Geometry: final body of the model. Coordinates: model frame, mm. A direction names the side the tool comes from. Give positions to 0.01 mm unless a question says otherwise; leave off trailing zeros. Loops run counter-clockwise (first coordinate to the right, second up) from the corner with the lowest first, then second, coordinate; pieces in that order, holes last. Notation, with made-up numbers: M 75,40 L 97,40 A13 ccw 97,60 Z; hole C 19.5,21.5 d10. An arc over 180 degrees is marked long. One line per question, with ' | ' between items. Start each with the question number.
Autodesk Inventor part; units mm, degrees
ref_plane "YZ Plane" through (0, 0, 0) normal (1, 0, 0) x (0, 1, 0)
ref_plane "XZ Plane" through (0, 0, 0) normal (0, 1, 0) x (-1, 0, 0)
ref_plane "XY Plane" through (0, 0, 0) normal (0, 0, 1) x (1, 0, 0)
sketch "Sketch1" plane through (0, 0, 0) normal (1, 0, 0) x (0, 1, 0)
  line L0 (-9.525, -87.3125) -> (9.525, -87.3125)
  line L1 (9.525, -87.3125) -> (9.525, 87.3125)
  line L2 (9.525, 87.3125) -> (-9.525, 87.3125)
  line L3 (-9.525, 87.3125) -> (-9.525, -87.3125)
  line L4 (-9.525, -87.3125) -> (9.525, 87.3125) construction
  line L5 (9.525, -87.3125) -> (-9.525, 87.3125) construction
  point P0 (0, 0)
  dimension "d0" = 19.05
  dimension "d1" = 174.625
extrude "Extrusion1" add sketch "Sketch1" along normal mid plane 9.525
sketch "Sketch2" plane through (4.7625, 0, 0) normal (1, 0, 0) x (0, 0, -1)
  line L0 (-100.0125, -3.175) -> (-74.6125, -3.175)
  line L1 (-74.6125, -3.175) -> (-74.6125, 3.175)
  line L2 (-74.6125, 3.175) -> (-100.0125, 3.175)
  line L3 (-100.0125, 3.175) -> (-100.0125, -3.175)
  line L4 (-87.3125, 9.525) -> (-87.3125, -9.525)
  line L5 (-100.0125, -3.175) -> (-74.6125, 3.175) construction
  line L6 (-74.6125, -3.175) -> (-100.0125, 3.175) construction
  point P0 (0, 0)
  point P1 (-87.3125, 0)
  point P2 (-87.3125, 3.175)
  point P3 (-87.3125, -3.175)
  dimension "d4" = 6.35
  dimension "d5" = 12.7
extrude "Extrusion2" cut sketch "Sketch2" against normal blind 25.4 contours L4 L2 L1 L0
sketch "Sketch3" plane through (-4.7625, 9.525, 87.3125) normal (0, 1, 0) x (1, 0, 0)
  line L0 (0, 0) -> (9.525, 0)
  circle A0 centre (4.7625, 4.7625) radius 2.6035
  point P0 (4.7625, 87.3125)
  point P1 (4.7625, 0)
  dimension "d8" = 5.207
  dimension "d9" = 4.7625
extrude "Extrusion3" cut sketch "Sketch3" against normal blind 6.35
sketch "Sketch4" plane through (4.7625, -3.175, 87.3125) normal (0, 1, 0) x (1, 0, 0)
  line L0 (-9.525, 0) -> (-9.525, 12.7)
  line L1 (0, 0) -> (-9.525, 0)
  line L2 (0, 12.7) -> (0, 0)
  line L3 (0, 12.7) -> (-9.525, 12.7)
  circle A0 centre (-4.7625, 4.7625) radius 2.6035
  circle A1 centre (-4.7625, 4.7625) radius 2.3813
  point P0 (-4.7625, 87.3125)
  dimension "d12" = 4.7625
extrude "Extrusion4" cut sketch "Sketch4" against normal blind 25.4 contours A1
properties part number "LongBraillePlunger"
Q1. Material intervals for L1, parallel to Z at x = 0, y = -7.25; L2, parallel to Z at x = 0, y = 5; L3, parallel to X at y = 5.25, z = 82.55, sorted ascending.
Q2. Section B-B, the plane x = 0. Output: boundary loops of the cut face in (y, z) (1 decimal), plus the area to 3 significant figures.
Q3. Draft query along X for faces 1 (the flat face through (0, 0, -87.312)), 2 (the cylindrical face through (-0.516, -6.306, 84.875)), 3 (the flat face through (-4.762, 0, 1)). Return one class per face: released by +X, released by -X, zero draft, split by the parting line, or undercut.
Q4. Set-up query: faces 4 (the cylindrical face through (-0.34, 6.39, 79.97)), 5 (the flat face through (0, 6, 87.312)), 6 (the flat face through (0, 3.175, 79)). Return all of +Z, -Z, +X, -X, +Y, -Y with unobstructed straight access to the full face (end or side cutting, diameter ignored); none if empty.
Q5. Section A-A, the plane z = 82.55. Output: boundary loops of the cut face in (x, y) (1 decimal), plus the area to 3 significant figures.
Q6. Section C-C, the plane y = 1.25. Output: boundary loops of the cut face in (x, z), plus the area to 3 significant figures.
Model answer:
1) L1: z = -87.31 to 80.17, 84.93 to 87.31 | L2: z = -87.31 to 79.95, 85.15 to 87.31 | L3: x = -4.76 to -2.6, 2.6 to 4.76
2) outline: M -9.5,-87.3 L 9.5,-87.3 L 9.5,79.9 L 3.2,79.9 L 3.2,74.6 L -3.2,74.6 L -3.2,80.2 L -9.5,80.2 Z; M -9.5,84.9 L -3.2,84.9 L -3.2,87.3 L -9.5,87.3 Z; M 3.2,85.2 L 9.5,85.2 L 9.5,87.3 L 3.2,87.3 Z | area: 3,180 mm^2
3) face 1: zero draft | face 2: undercut | face 3: released by -X
4) face 4: +Y | face 5: +Z, +X, -X, +Y, -Y | face 6: +Z, +X, -X
5) outline: M -4.8,-9.5 L -2.4,-9.5 L -2.4,-3.2 L -4.8,-3.2 Z; M -4.8,3.2 L -2.6,3.2 L -2.6,9.5 L -4.8,9.5 Z; M 2.4,-9.5 L 4.8,-9.5 L 4.8,-3.2 L 2.4,-3.2 Z; M 2.6,3.2 L 4.8,3.2 L 4.8,9.5 L 2.6,9.5 Z | area: 57.7 mm^2
6) outline: M -4.76,-87.31 L 4.76,-87.31 L 4.76,74.61 L -4.76,74.61 Z | area: 1,540 mm^2
